from build123d import *

# Parameters (mm, degrees)
EXTRUDE_1_DEPTH             = 90
SKETCH_2_W                  = 90
SKETCH_2_H                  = 17.75
EXTRUDE_2_DEPTH             = 8.2
SKETCH_3_W                  = 90
SKETCH_3_H                  = 102.45
EXTRUDE_3_DEPTH             = 8.2
SKETCH_4_W                  = 3.95
SKETCH_4_H                  = 2.25
CUT_EXTRUDE_1_DEPTH         = 91
SKETCH_5_W                  = 3.95
SKETCH_5_H                  = 29.5
CUT_EXTRUDE_2_DEPTH         = 91
SKETCH_6_W                  = 3.95
SKETCH_6_H                  = 9
CUT_EXTRUDE_3_DEPTH         = 91
SKETCH_7_W                  = 3.95
SKETCH_7_H                  = 29.5
CUT_EXTRUDE_4_DEPTH         = 91
SKETCH_8_W                  = 3.95
SKETCH_8_H                  = 6.2
CUT_EXTRUDE_5_DEPTH         = 91
SKETCH_9_W                  = 2.25
SKETCH_9_H                  = 3.95
CUT_EXTRUDE_6_DEPTH         = 91
SKETCH_10_W                 = 4.5
SKETCH_10_H                 = 3.95
CUT_EXTRUDE_7_DEPTH         = 91
SKETCH_11_W                 = 2.25
SKETCH_11_H                 = 3.95
CUT_EXTRUDE_8_DEPTH         = 91
SKETCH_12_W                 = 19.6
SKETCH_12_H                 = 96.1
CUT_EXTRUDE_9_DEPTH         = 86.2
HOLE_WIZARD_4_5_4_5_1_D     = 4.5
HOLE_WIZARD_4_5_4_5_1_DEPTH = 90
HOLE_WIZARD_2_5_2_5_1_D     = 2.5
HOLE_WIZARD_2_5_2_5_1_DEPTH = 90
SKETCH_20_R                 = 1.649948342
SKETCH_20_R_2               = 1.660581376
SKETCH_20_R_3               = 1.430745594
SKETCH_20_R_4               = 1.573250385
SKETCH_20_R_5               = 1.502029841
SKETCH_20_R_6               = 1.53795619
EXTRUDE_5_DEPTH             = 90


with BuildPart() as part:
    # Эскиз1 → Бобышка-Вытянуть1 (new body)
    with BuildSketch(Plane(origin=(90, 0, 0), x_dir=(0, 0, -1), z_dir=(1, 0, 0))):
        with BuildLine():
            Line((6.75, 40.906238208), (6.75, 135.75))
            Line((6.75, 135.75), (-11.593761792, 135.75))
            ThreePointArc((-11.593761792, 135.75), (-15.325, 134.5), (-11.593761793, 133.25))
            Line((-11.593761793, 133.25), (-11, 133.25))
            Line((-11, 133.25), (-11, 99.75))
            Line((-11, 99.75), (-11.593761792, 99.75))
            ThreePointArc((-11.593761792, 99.75), (-15.325, 98.5), (-11.593761792, 97.25))
            Line((-11.593761792, 97.25), (-11, 97.25))
            Line((-11, 97.25), (-11, 84.25))
            Line((-11, 84.25), (-11.593761792, 84.25))
            ThreePointArc((-11.593761792, 84.25), (-15.325, 83), (-11.593761792, 81.75))
            Line((-11.593761792, 81.75), (-11, 81.75))
            Line((-11, 81.75), (-11, 48.25))
            Line((-11, 48.25), (-11.593761792, 48.25))
            ThreePointArc((-11.593761792, 48.25), (-15.325, 47), (-11.593761792, 45.75))
            Line((-11.593761792, 45.75), (-11, 45.75))
            Line((-11, 45.75), (-11, 41.5))
            Line((-11, 41.5), (-6.75, 41.5))
            Line((-6.75, 41.5), (-6.75, 40.906238208))
            ThreePointArc((-6.75, 40.906238208), (-5.5, 37.175), (-4.25, 40.906238208))
            Line((-4.25, 40.906238208), (-4.25, 41.5))
            Line((-4.25, 41.5), (4.25, 41.5))
            Line((4.25, 41.5), (4.25, 40.906238208))
            ThreePointArc((4.25, 40.906238208), (5.5, 37.175), (6.75, 40.906238208))
        make_face()
    extrude(amount=-EXTRUDE_1_DEPTH)

    # Эскиз2 → Бобышка-Вытянуть2 (add)
    with BuildSketch(Plane(origin=(0, 135.75, 0), x_dir=(-1, 0, 0), z_dir=(0, 1, 0))):
        with Locations((-45, 2.125)):
            Rectangle(SKETCH_2_W, SKETCH_2_H)
    extrude(amount=EXTRUDE_2_DEPTH)

    # Эскиз3 → Бобышка-Вытянуть3 (add)
    with BuildSketch(Plane(origin=(0, 0, -6.75), x_dir=(-1, 0, 0), z_dir=(0, 0, -1))):
        with Locations((-45, 92.725)):
            Rectangle(SKETCH_3_W, SKETCH_3_H)
    extrude(amount=EXTRUDE_3_DEPTH)

    # Эскиз4 → Вырез-Вытянуть1 (cut, through all)
    with BuildSketch(Plane.ZY):
        with Locations((-12.975, 42.625)):
            Rectangle(SKETCH_4_W, SKETCH_4_H)
    extrude(amount=-CUT_EXTRUDE_1_DEPTH, mode=Mode.SUBTRACT)

    # Эскиз5 → Вырез-Вытянуть2 (cut, through all)
    with BuildSketch(Plane.ZY):
        with Locations((-12.975, 65)):
            Rectangle(SKETCH_5_W, SKETCH_5_H)
    extrude(amount=-CUT_EXTRUDE_2_DEPTH, mode=Mode.SUBTRACT)

    # Эскиз6 → Вырез-Вытянуть3 (cut, through all)
    with BuildSketch(Plane.ZY):
        with Locations((-12.975, 90.75)):
            Rectangle(SKETCH_6_W, SKETCH_6_H)
    extrude(amount=-CUT_EXTRUDE_3_DEPTH, mode=Mode.SUBTRACT)

    # Эскиз7 → Вырез-Вытянуть4 (cut, through all)
    with BuildSketch(Plane.ZY):
        with Locations((-12.975, 116.5)):
            Rectangle(SKETCH_7_W, SKETCH_7_H)
    extrude(amount=-CUT_EXTRUDE_4_DEPTH, mode=Mode.SUBTRACT)

    # Эскиз8 → Вырез-Вытянуть5 (cut, through all)
    with BuildSketch(Plane.ZY):
        with Locations((-12.975, 140.85)):
            Rectangle(SKETCH_8_W, SKETCH_8_H)
    extrude(amount=-CUT_EXTRUDE_5_DEPTH, mode=Mode.SUBTRACT)

    # Эскиз9 → Вырез-Вытянуть6 (cut, through all)
    with BuildSketch(Plane.ZY):
        with Locations((-9.875, 141.975)):
            Rectangle(SKETCH_9_W, SKETCH_9_H)
    extrude(amount=-CUT_EXTRUDE_6_DEPTH, mode=Mode.SUBTRACT)

    # Эскиз10 → Вырез-Вытянуть7 (cut, through all)
    with BuildSketch(Plane.ZY):
        with Locations((0, 141.975)):
            Rectangle(SKETCH_10_W, SKETCH_10_H)
    extrude(amount=-CUT_EXTRUDE_7_DEPTH, mode=Mode.SUBTRACT)

    # Эскиз11 → Вырез-Вытянуть8 (cut, through all)
    with BuildSketch(Plane.ZY):
        with Locations((9.875, 141.975)):
            Rectangle(SKETCH_11_W, SKETCH_11_H)
    extrude(amount=-CUT_EXTRUDE_8_DEPTH, mode=Mode.SUBTRACT)

    # Эскиз12 → Вырез-Вытянуть9 (cut)
    with BuildSketch(Plane(origin=(90, 0, 0), x_dir=(0, 0, -1), z_dir=(1, 0, 0))):
        with Locations((0, 90.75)):
            Rectangle(SKETCH_12_W, SKETCH_12_H)
    extrude(amount=-CUT_EXTRUDE_9_DEPTH, mode=Mode.SUBTRACT)

    # Диаметр отверстия Ø4.5 (4.5)1
    with Locations(Plane.ZY):
        with Locations((-13.25, 47), (-13.25, 83), (-13.25, 98.5), (-13.25, 134.5), (-5.5, 142.25), (5.5, 142.25)):
            Hole(HOLE_WIZARD_4_5_4_5_1_D / 2, depth=HOLE_WIZARD_4_5_4_5_1_DEPTH)

    # Диаметр отверстия Ø2.5 (2.5)1
    with Locations(Plane(origin=(90, 0, 0), x_dir=(0, 0, -1), z_dir=(1, 0, 0))):
        with Locations((-13.25, 98.5), (-13.25, 134.5), (-13.25, 47), (-13.25, 83), (5.5, 39.25), (-5.5, 39.25)):
            Hole(HOLE_WIZARD_2_5_2_5_1_D / 2, depth=HOLE_WIZARD_2_5_2_5_1_DEPTH)

    # Эскиз20 → Бобышка-Вытянуть5 (add)
    with BuildSketch(Plane(origin=(90, 0, 0), x_dir=(0, 0, -1), z_dir=(1, 0, 0))):
        with Locations((-13.25, 134.5)):
            Circle(SKETCH_20_R)
        with Locations((-13.25, 98.5)):
            Circle(SKETCH_20_R_2)
        with Locations((-13.25, 83)):
            Circle(SKETCH_20_R_3)
        with Locations((-13.25, 47)):
            Circle(SKETCH_20_R_4)
        with Locations((-5.5, 39.25)):
            Circle(SKETCH_20_R_5)
        with Locations((5.5, 39.25)):
            Circle(SKETCH_20_R_6)
    extrude(amount=-EXTRUDE_5_DEPTH)


solid = part.part
For this review, take the finished solid that the model builds, in its own axes (mm). A direction names the side the tool comes from. Round coordinates to 2 decimals unless told otherwise and drop trailing zeros. Write each loop counter-clockwise with the first axis right and the second up, starting at its lowest first coordinate (ties: lowest second). Pieces come first, ordered by that corner, then holes. Notation, with made-up numbers: (88.5, -21.5) - (123.5, -21.5) arc R11 ccw to (123.5, -16.5) - close; hole circle Ø8 at (69, 10). An arc over 180 degrees is marked (long way). Write item = value, one per line. Start each with the question number.
1. Consider section D-D on z = 5.5. State the section outline as (x, y) points (3 decimals), plus the area to 3 significant figures.
2. Consider section A-A on z = 13.25. State the section outline as (x, y) points (3 decimals), plus the area to 3 significant figures.
3. Consider section B-B on y = 39.25. State the section outline as (x, z) points (3 decimals), plus the area to 3 significant figures.
4. Consider section C-C on y = 130. State the section outline as (x, z) points.
5. For faces 4 (the face through (44, 140, 10)), 5 (the face through (46, 44, 11)), 6 (the face through (3.8, 91, 0)), 7 (the face through (46, 138, 11)), 8 (the face through (46, 41.5, -9)), list the 3-axis set-ups (+Z, -Z, +X, -X, +Y, -Y) from which the entire face can be reached by the end or side of a thin tool; tool diameter is ignored.
6. For pin 1 Ø1.5 at (y, z) = (133, 4.5) entering from -X; pin 2 Ø0.5 at (x, z) = (60, 11.5) entering from +Y; pin 3 Ø4 at (x, z) = (60.5, 11.5) entering from +Y; pin 4 Ø6.5 at (x, y) = (48.5, 92.5) entering from +Z, all flat-tipped, find the tip position at first contact; note any pin that passes through.
7. Wall thickness on L1, parallel to Z at x = 34, y = 142; L2, parallel to Y at x = 74, z = 11.5; L3, parallel to Z at x = 42, y = 134.5 (3 decimals): over which ranges is each line inside the solid? List them lowest first.
8. Draft analysis for pull direction Z (two halves, no side actions). For faces 1 (the face through (44, 95.25, -13)), 2 (the face through (45.63, 37.176, -5.428)), 3 (the face through (44, 43, -11)), state which applies: released by +Z, released by -Z, zero draft, split by the parting line, or undercut.
Evaluation:
q1.outline = (0, 37.175) - (90, 37.175) - (90, 42.7) - (3.8, 42.7) - (3.8, 138.8) - (90, 138.8) - (90, 140) - (0, 140) - close
q1.area = 970 mm2
q2.outline = (0, 44.925) - (90, 44.925) - (90, 49.075) - (0, 49.075) - close; (0, 80.925) - (90, 80.925) - (90, 85.075) - (0, 85.075) - close; (0, 96.425) - (90, 96.425) - (90, 100.575) - (0, 100.575) - close; (0, 132.425) - (90, 132.425) - (90, 136.575) - (0, 136.575) - close
q2.area = 1,490 mm2
q3.outline = (0, -7.575) - (90, -7.575) - (90, -3.425) - (0, -3.425) - close; (0, 3.425) - (90, 3.425) - (90, 7.575) - (0, 7.575) - close
q3.area = 747 mm2
q4.outline = (0, -11) - (90, -11) - (90, -9.8) - (3.8, -9.8) - (3.8, 9.8) - (90, 9.8) - (90, 11) - (0, 11) - close
q5.face_4 = +Z, +X, -X, +Y
q5.face_5 = +X, -X, -Y
q5.face_6 = +X
q5.face_7 = +X, -X, +Y
q5.face_8 = -Z, +X, -X
q6.pin_1 = 0
q6.pin_2 = 135.93
q6.pin_3 = 140
q6.pin_4 = 11
q7.L1 = -8.75 to -7.74, -3.26 to -2.25, 2.25 to 3.26, 7.74 to 8.75
q7.L2 = 45.75 to 48.25, 81.75 to 84.25, 97.25 to 99.75, 133.25 to 135.75
q7.L3 = -11 to -9.8, 9.8 to 15.325
q8.face_1 = zero draft
q8.face_2 = undercut
q8.face_3 = released by -Z
